Geometry check sheet. Reference: the model listing, model coordinates, mm. A direction names the side the tool comes from. Give positions to 0.01 mm unless a question says otherwise; leave off trailing zeros. Write each loop counter-clockwise with the first axis right and the second up, starting at its lowest first coordinate (ties: lowest second). Pieces come first, ordered by that corner, then holes. Notation, with made-up numbers: (-18, -8.5) - (20, -8.5) arc R27 ccw to (20, 9.5) - close; hole circle Ø1 at (50, 59.5). An arc over 180 degrees is marked (long way). Use a Markdown table: item, result.
```python
from build123d import *

# Parameters (mm, degrees)
SKETCH1_R                       = 3.175
BOSS_EXTRUDE1_DEPTH             = 3.81
FILLET1_R                       = 5.08
SKETCH3_R                       = 3.175
CUT_EXTRUDE2_DEPTH              = 8.62
BOSS_EXTRUDE2_DEPTH             = 6.35
SKETCH6_R                       = 2.286
CUT_EXTRUDE3_DEPTH              = 6.35
BOSS_EXTRUDE3_DEPTH             = 5.08
FILLET2_R                       = 1.905
FILLET3_R                       = 1.905
BOSS_EXTRUDE4_REACH             = 8.35
BOSS_EXTRUDE4_DIRECTION_2_REACH = 9.62


with BuildPart() as part:
    # Sketch1 → Boss-Extrude1 (new body, symmetric)
    with BuildSketch(Plane(origin=(0, 0, 0), x_dir=(1, 0, 0), z_dir=(0, 1, 0))):
        with BuildLine():
            Line((-43.270256121, 34.29), (-4.490128061, -4.490128061))
            Line((-4.490128061, -4.490128061), (6.35, -10.668))
            Line((6.35, -10.668), (57.15, -10.668))
            Line((57.15, -10.668), (57.15, 6.35))
            Line((57.15, 6.35), (20.590768363, 6.35))
            Line((20.590768363, 6.35), (-7.349231637, 34.29))
            ThreePointArc((-7.349231637, 34.29), (-25.309743879, 52.250512242), (-43.270256121, 34.29))
        make_face()
        Circle(SKETCH1_R, mode=Mode.SUBTRACT)
    extrude(amount=BOSS_EXTRUDE1_DEPTH, both=True)

    # Fillet1
    fillet1_edges = [part.edges().sort_by_distance(p)[0] for p in [
        (-43.270256121, 0, -34.29),
        (20.590768363, 0, -6.35),
        (57.15, 0, -6.35),
        (6.35, 0, 10.668),
    ]]
    fillet(fillet1_edges, radius=FILLET1_R)

    # Sketch3 → Cut-Extrude2 (cut, through all)
    with BuildSketch(Plane(origin=(0, 3.81, 0), x_dir=(1, 0, 0), z_dir=(0, 1, 0))):
        with Locations((-25.309743879, 41.91)):
            Circle(SKETCH3_R)
    extrude(amount=-CUT_EXTRUDE2_DEPTH, mode=Mode.SUBTRACT)

    # Sketch4 → Boss-Extrude2 (add)
    with BuildSketch(Plane(origin=(0, 3.81, 0), x_dir=(1, 0, 0), z_dir=(0, 1, 0))):
        with BuildLine():
            Line((57.15, -10.668), (7.695948183, -10.668))
            ThreePointArc((7.695948183, -10.668), (6.394891779, -10.498565368), (5.180624356, -10.001563871))
            Line((5.180624356, -10.001563871), (5.180624356, -4.318))
            ThreePointArc((5.180624356, -4.318), (7.040496295, 0.172128061), (11.530624356, 2.032))
            Line((11.530624356, 2.032), (57.15, 2.032))
            Line((57.15, 2.032), (57.15, -10.668))
        make_face()
    extrude(amount=BOSS_EXTRUDE2_DEPTH)

    # Sketch6 → Cut-Extrude3 (cut)
    with BuildSketch(Plane.XY.offset(10.668)):
        with Locations((15.315948183, 6.35)):
            Circle(SKETCH6_R)
        with Locations((50.875948183, 6.35)):
            Circle(SKETCH6_R)
    extrude(amount=-CUT_EXTRUDE3_DEPTH, mode=Mode.SUBTRACT)

    # Sketch7 → Boss-Extrude3 (add)
    with BuildSketch(Plane.XY.offset(10.668)):
        with BuildLine():
            Line((57.15, 10.16), (7.695948183, 10.16))
            Line((7.695948183, 10.16), (7.695948183, 4.318))
            Line((7.695948183, 4.318), (12.876357848, 4.318))
            ThreePointArc((12.876357848, 4.318), (14.235456237, 9.335491945), (18.490948183, 6.35))
            ThreePointArc((18.490948183, 6.35), (18.301440128, 5.269508055), (17.755538517, 4.318))
            Line((17.755538517, 4.318), (48.436357848, 4.318))
            ThreePointArc((48.436357848, 4.318), (49.795456237, 9.335491945), (54.050948183, 6.35))
            ThreePointArc((54.050948183, 6.35), (53.861440128, 5.269508055), (53.315538517, 4.318))
            Line((53.315538517, 4.318), (57.15, 4.318))
            Line((57.15, 4.318), (57.15, 10.16))
        make_face()
    extrude(amount=BOSS_EXTRUDE3_DEPTH)

    # Fillet2
    fillet2_edges = [part.edges().sort_by_distance(p)[0] for p in [
        (53.315538517, 4.318, 13.208),
        (12.876357848, 4.318, 13.208),
        (17.755538517, 4.318, 13.208),
        (48.436357848, 4.318, 13.208),
    ]]
    fillet(fillet2_edges, radius=FILLET2_R)

    # Fillet3
    fillet3_edges = [part.edges().sort_by_distance(p)[0] for p in [
        (34.31157461, 3.81, -2.032),
        (7.040496295, 3.81, -0.172128061),
        (5.180624356, 3.81, 7.159781936),
    ]]
    fillet(fillet3_edges, radius=FILLET3_R)

    # Boss-Extrude4: up to this face of the body (flat: up to its plane)
    boss_extrude4_end = Plane(part.part.faces().sort_by_distance((31.766522001, 10.16, 6.837548853))[0])
    # Sketch8 → Boss-Extrude4 (add, up to the picked face)
    with BuildSketch(Plane(origin=(0, 3.81, 0), x_dir=(1, 0, 0), z_dir=(0, 1, 0)), mode=Mode.PRIVATE) as boss_extrude4_sk1:
        with BuildLine():
            Line((5.180624356, -15.748), (7.695948183, -15.748))
            Line((7.695948183, -15.748), (7.695948183, -10.668))
            ThreePointArc((7.695948183, -10.668), (6.394891779, -10.498565368), (5.180624356, -10.001563871))
            Line((5.180624356, -10.001563871), (5.180624356, -15.748))
        make_face()
    boss_extrude4_tool1 = split(extrude(boss_extrude4_sk1.sketch, amount=BOSS_EXTRUDE4_REACH, mode=Mode.PRIVATE), bisect_by=boss_extrude4_end, keep=Keep.BOTH, mode=Mode.PRIVATE)
    add(boss_extrude4_tool1.solids().sort_by_distance((6.412294, 3.81, 13.096367))[0])

    # Boss-Extrude4 direction 2: up to this face of the body (flat: up to its plane)
    boss_extrude4_direction_2_end = Plane(part.part.faces().sort_by_distance((1.392944323, -3.81, -15.281162376))[0])
    # Sketch8 → Boss-Extrude4 direction 2 (add, up to the picked face)
    with BuildSketch(Plane(origin=(0, 3.81, 0), x_dir=(1, 0, 0), z_dir=(0, 1, 0)), mode=Mode.PRIVATE) as boss_extrude4_direction_2_sk1:
        with BuildLine():
            Line((5.180624356, -15.748), (7.695948183, -15.748))
            Line((7.695948183, -15.748), (7.695948183, -10.668))
            ThreePointArc((7.695948183, -10.668), (6.394891779, -10.498565368), (5.180624356, -10.001563871))
            Line((5.180624356, -10.001563871), (5.180624356, -15.748))
        make_face()
    boss_extrude4_direction_2_tool1 = split(extrude(boss_extrude4_direction_2_sk1.sketch, amount=-BOSS_EXTRUDE4_DIRECTION_2_REACH, mode=Mode.PRIVATE), bisect_by=boss_extrude4_direction_2_end, keep=Keep.BOTH, mode=Mode.PRIVATE)
    add(boss_extrude4_direction_2_tool1.solids().sort_by_distance((6.412294, 3.81, 13.096367))[0])


solid = part.part
```
1) Set-up check for faces 1 (the flat face through (38, 0, -6.35)), 2 (the cylindrical face through (6.99, 7.91, -0.12)), 3 (the flat face through (5.181, 5, 11)), 4 (the flat face through (33, 4.318, 13)): record each of +Z, -Z, +X, -X, +Y, -Y from which the full face is reachable in a straight line by a thin tool's end or side.
Working result:
| item | result |
|---|---|
| face 1 | -Z, +X, +Y, -Y |
| face 2 | -Z, -X, +Y |
| face 3 | +Z, -X, +Y |
| face 4 | +Z, +X, -Y |
2) Material ranges on L1, parallel to Z at x = 43, y = -2.75; L2, parallel to Y at x = -32, z = -34; L3, parallel to X at y = -1.25, z = -40, recorded low to high. Write a range as from..to.
Working result:
| item | result |
|---|---|
| L1 | z = -6.35..10.67 |
| L2 | y = -3.81..3.81 |
| L3 | x = -42.34..-27.85, -22.77..-8.28 |
3) Section check C-C on x = 39.5. Record the boundary of the cut face in (y, z) (3 decimals).
Working result:
| item | result |
|---|---|
| outline | (-3.81, -6.35) - (3.81, -6.35) - (3.81, -3.937) arc R1.905 cw to (5.715, -2.032) - (10.16, -2.032) - (10.16, 15.748) - (4.318, 15.748) - (4.318, 10.668) - (-3.81, 10.668) - close |
4) Section check D-D on x = 0. Record the boundary of the cut face in (y, z) (3 decimals).
Working result:
| item | result |
|---|---|
| outline | (-3.81, -26.941) - (3.81, -26.941) - (3.81, -3.175) - (-3.81, -3.175) - close; (-3.81, 3.175) - (3.81, 3.175) - (3.81, 7.049) - (-3.81, 7.049) - close |
5) Section check B-B on z = -41.91. Record the boundary of the cut face in (x, y), then the cut area to 3 significant figures.
Working result:
| item | result |
|---|---|
| outline | (-41.57, -3.81) - (-28.48, -3.81) - (-28.48, 3.81) - (-41.57, 3.81) - close; (-22.13, -3.81) - (-9.05, -3.81) - (-9.05, 3.81) - (-22.13, 3.81) - close |
| area | 199 mm² |
6) Mould release check, pull along Y, two halves, no side actions. Record for faces 5 (the cylindrical face through (48.592, 6.451, 7.537)), 6 (the cylindrical face through (-26, 0.05, -38.81)), 7 (the cylindrical face through (34.63, 4.38, -2.58)): pulls with the +Y half, pulls with the -Y half, needs draft (parallel to the pull), parting line crosses it, or undercut.
Working result:
| item | result |
|---|---|
| face 5 | undercut |
| face 6 | needs draft |
| face 7 | pulls with the +Y half |
7) Section check A-A on y = 1.75. Record the boundary of the cut face in (x, z) (3 decimals), then the cut area to 3 significant figures.
Working result:
| item | result |
|---|---|
| outline | (-43.062, -37.016) arc R17.961 ccw to (-7.349, -34.29) - (19.103, -7.838) arc R5.08 cw to (22.695, -6.35) - (52.07, -6.35) arc R5.08 ccw to (57.15, -1.27) - (57.15, 10.668) - (7.696, 10.668) - (7.696, 15.748) - (5.181, 15.748) - (5.181, 10.002) - (-4.49, 4.49) - (-41.633, -32.653) arc R5.08 ccw to start; hole circle Ø6.35 at (-25.31, -41.91); hole circle Ø6.35 at (0, 0) |
| area | 2,530 mm² |
8) Depth check by flat-ended pin: P1, Ø2.5, axis at x = 42.5, y = 1.5, coming from the -Z side; P2, Ø1.3, axis at x = 9, z = 13, coming from the -Y side; P3, Ø1.5, axis at x = 7, y = 7.5, coming from the -Z side; P4, Ø10, axis at x = -2, z = 0.5, coming from the -Y side. Enter the tip coordinate at first touch or a pass-through.
Working result:
| item | result |
|---|---|
| P1 | stops at z = -6.35 |
| P2 | stops at y = 4.32 |
| P3 | stops at z = -0.78 |
| P4 | stops at y = -3.81 |
